```python
from build123d import *

# Parameters (mm, degrees)
SKETCH1_R           = 10
BOSS_EXTRUDE1_DEPTH = 0.5
SKETCH2_R           = 10
BOSS_EXTRUDE2_DEPTH = 0.5
SKETCH3_R           = 10
BOSS_EXTRUDE3_DEPTH = 1
SKETCH5_R           = 1.6
CUT_EXTRUDE2_DEPTH  = 3
SKETCH8_R           = 1.6
CUT_EXTRUDE4_DEPTH  = 10
FILLET1_R           = 0.4
SKETCH9_R           = 4.5
SKETCH9_R_2         = 3.5
BOSS_EXTRUDE4_DEPTH = 3
SKETCH10_R          = 3.5
CUT_EXTRUDE5_DEPTH  = 1
FILLET3_R           = 1.2


with BuildPart() as part:
    # Sketch1 → Boss-Extrude1 (new body)
    with BuildSketch(Plane(origin=(0, 0, 0), x_dir=(1, 0, 0), z_dir=(0, 1, 0))):
        Circle(SKETCH1_R)
    extrude(amount=BOSS_EXTRUDE1_DEPTH)

    # Sketch2 → Boss-Extrude2 (add)
    with BuildSketch(Plane(origin=(0, 0.5, 0), x_dir=(1, 0, 0), z_dir=(0, 1, 0))):
        Circle(SKETCH2_R)
    extrude(amount=BOSS_EXTRUDE2_DEPTH)

    # Sketch3 → Boss-Extrude3 (add)
    with BuildSketch(Plane(origin=(0, 1, 0), x_dir=(1, 0, 0), z_dir=(0, 1, 0))):
        Circle(SKETCH3_R)
    extrude(amount=BOSS_EXTRUDE3_DEPTH)

    # Sketch5 → Cut-Extrude2 (cut, through all)
    with BuildSketch(Plane(origin=(0, 2, 0), x_dir=(1, 0, 0), z_dir=(0, 1, 0))):
        Circle(SKETCH5_R)
    extrude(amount=-CUT_EXTRUDE2_DEPTH, mode=Mode.SUBTRACT)

    # Sketch8 → Cut-Extrude4 (cut)
    with BuildSketch(Plane(origin=(0, 2, 0), x_dir=(1, 0, 0), z_dir=(0, 1, 0))):
        with Locations((-6.8, 0)):
            Circle(SKETCH8_R)
        with Locations((6.8, 0)):
            Circle(SKETCH8_R)
        with Locations((0, 6.8)):
            Circle(SKETCH8_R)
        with Locations((0, -6.8)):
            Circle(SKETCH8_R)
    extrude(amount=-CUT_EXTRUDE4_DEPTH, mode=Mode.SUBTRACT)

    # Fillet1
    fillet1_edges = [part.edges().sort_by_distance(p)[0] for p in [
        (-10, 0, 0),
        (-10, 2, 0),
    ]]
    fillet(fillet1_edges, radius=FILLET1_R)

    # Sketch9 → Boss-Extrude4 (add)
    with BuildSketch(Plane.XZ):
        Circle(SKETCH9_R)
        Circle(SKETCH9_R_2, mode=Mode.SUBTRACT)
    extrude(amount=BOSS_EXTRUDE4_DEPTH)

    # Sketch10 → Cut-Extrude5 (cut)
    with BuildSketch(Plane.XZ):
        Circle(SKETCH10_R)
    extrude(amount=-CUT_EXTRUDE5_DEPTH, mode=Mode.SUBTRACT)

    # Fillet3
    fillet3_edges = [part.edges().sort_by_distance(p)[0] for p in [
        (-3.5, 1, 0),
    ]]
    fillet(fillet3_edges, radius=FILLET3_R)


solid = part.part
```
Geometry: final body of the model. Coordinates: model frame, mm. A direction names the side the tool comes from. Coordinates: 2 decimals unless noted, no trailing zeros. Loops run counter-clockwise (first coordinate to the right, second up) from the corner with the lowest first, then second, coordinate; pieces in that order, holes last. Notation, with made-up numbers: (54, 84) -> (59, 84) arc R11 cw to (59, 95) -> close; hole circle Ø1 at (2.5, 12.5). An arc over 180 degrees is marked (long way). Use a Markdown table: item, result. Add a question column.
(1) Line query: line 1 along X through (y, z) = (1.55, 0); line 2 along Y through (x, z) = (7.5, -1.5). Output: solid intervals per line, ascending.
(2) Pin query (flat end, axial travel): pin 1 Ø2 at (x, y) = (5, 1) entering from -Z; pin 2 Ø3.5 at (x, z) = (-6.8, 0) entering from -Y; pin 3 Ø2 at (y, z) = (-0.5, -3) entering from +X. Return the tip coordinate at first contact, or that it passes through.
(3) Access query for faces 1 (the flat face through (4.1, 0, -2.3)), 2 (the cylindrical face through (-0.35, 1.01, -5.24)). Directions: +Z, -Z, +X, -X, +Y, -Y. A direction counts if a zero-diameter tool reaches every point of the face in a straight line with its end or side. Return the directions, or none.
(4) Section query A-A, the plane z = 0. State how many separate pieces and enclosed holes the cut face has, plus the area to 3 significant figures.
(5) Section query C-C, the plane y = -2.6. Return loops of the section in (x, z), plus the area to 3 significant figures.
(6) Mould query, pull axis Z, two halves, no side actions, for faces 3 (the cylindrical face through (-2.17, 0.99, 9.76)), 4 (the flat face through (0, 2, 2)), 5 (the cylindrical face through (8.28, 1.01, 0.61)), 6 (the flat face through (0, 1, 2)). Classes: pulls with the +Z half, pulls with the -Z half, needs draft (parallel to the pull), parting line crosses it, or undercut.
Answer:
| question | item | result |
|---|---|---|
| 1 | line 1 | x = -10 to -8.4, -5.2 to -1.6, 1.6 to 5.2, 8.4 to 10 |
| 1 | line 2 | y = 0 to 2 |
| 2 | pin 1 | stops at z = -9.17 |
| 2 | pin 2 | stops at y = 0 |
| 2 | pin 3 | stops at x = 9.7 |
| 3 | face 1 | -Y |
| 3 | face 2 | +Y, -Y |
| 4 | separate pieces | 4 |
| 4 | enclosed holes | 0 |
| 4 | area | 23.5 mm^2 |
| 5 | outline | circle Ø9 at (0, 0); hole circle Ø7 at (0, 0) |
| 5 | area | 25.1 mm^2 |
| 6 | face 3 | parting line crosses it |
| 6 | face 4 | needs draft |
| 6 | face 5 | undercut |
| 6 | face 6 | undercut |
